Can you work these out from the drawing? Everything is in mm from the part's minimum corner. Round coordinates to 2 decimals unless told otherwise and drop trailing zeros. Loops run counter-clockwise (first coordinate to the right, second up) from the corner with the lowest first, then second, coordinate; pieces in that order, holes last. Notation, with made-up numbers: M 46,-9.75 L 51,-9.75 A16 cw 51,13.25 Z; hole C 46,-33 d9. An arc over 180 degrees is marked long. Use a Markdown table: item, result.
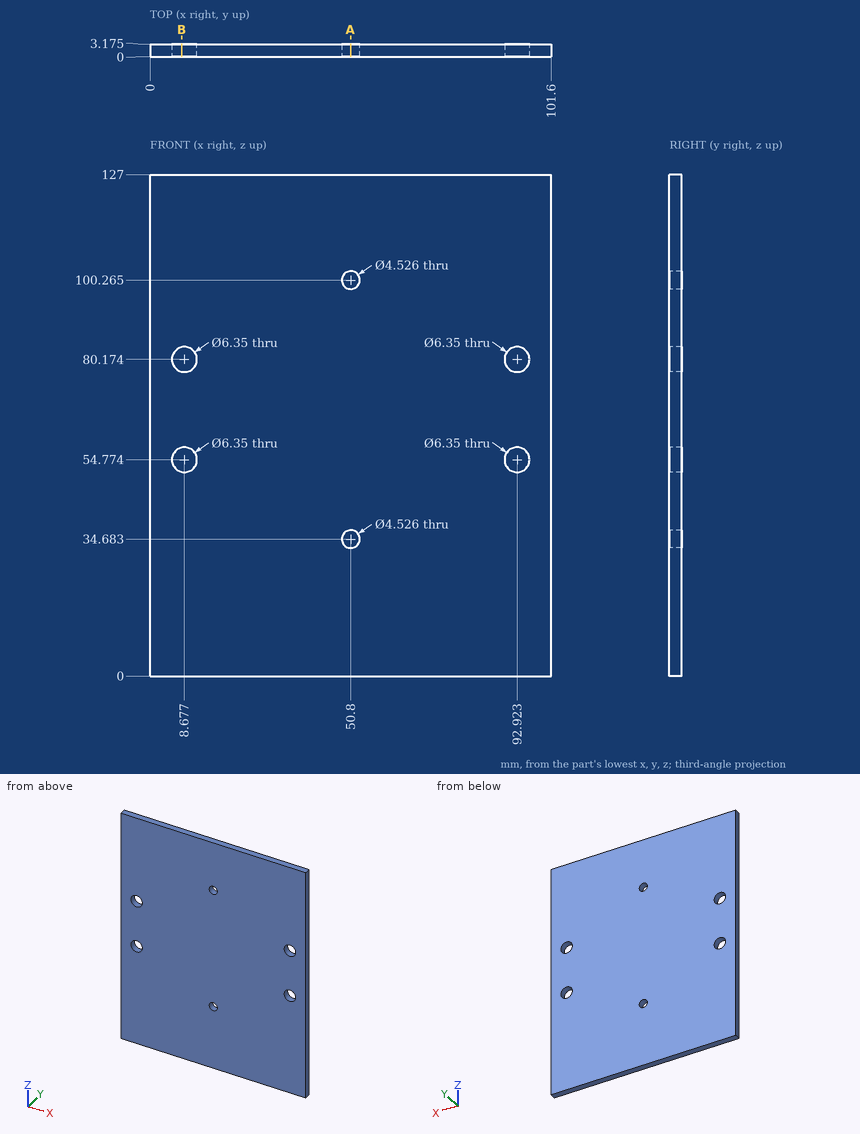
1. Imagine slicing it at B-B, the plane x = 8. Write out the boundary of the cut face in (y, z) (1 decimal).
Answer sheet:
| item | result |
|---|---|
| outline | M 0,0 L 3.2,0 L 3.2,51.7 L 0,51.7 Z; M 0,57.9 L 3.2,57.9 L 3.2,77.1 L 0,77.1 Z; M 0,83.3 L 3.2,83.3 L 3.2,127 L 0,127 Z |
2. I need wall thicknesses on probe 1 along Z at (x, y) = (50.8, 1.95) (1 decimal); probe 2 along X at (y, z) = (1.85, 55); probe 3 along Z at (x, y) = (93.5, 0.55) (1 decimal). Which ranges of each line are inside material? Lowest first, please. Write a range as from..to.
Answer sheet:
| item | result |
|---|---|
| probe 1 | 0..32.4, 36.9..98, 102.5..127 |
| probe 2 | 0..5.51, 11.84..89.76, 96.09..101.6 |
| probe 3 | 0..51.7, 57.9..77.1, 83.3..127 |
3. Imagine slicing it at A-A, the plane x = 50.8. Write out the boundary of the cut face in (y, z) (1 decimal).
Answer sheet:
| item | result |
|---|---|
| outline | M 0,0 L 3.2,0 L 3.2,32.4 L 0,32.4 Z; M 0,36.9 L 3.2,36.9 L 3.2,98 L 0,98 Z; M 0,102.5 L 3.2,102.5 L 3.2,127 L 0,127 Z |
4. For pin 1 Ø2.5 at (x, z) = (50.8, 34.68) entering from +Y, with a flat end and sliding along its axis, tell me the tip position at first contact or that it passes through.
Answer sheet:
| item | result |
|---|---|
| pin 1 | through |
